Verification items for the finished model (mm, model axes). Give positions to 0.01 mm unless a question says otherwise; leave off trailing zeros. Order: outer loops, then holes, each group sorted by start corner. A loop starts at its lowest first (then second) coordinate and runs counter-clockwise, first axis right, second up. Notation, with made-up numbers: M 34,-12 L 40,-12 A6 ccw 40,-7 Z; hole C 56.25,-22 d7. An arc over 180 degrees is marked long. Answer as a JSON object with one key per item and string values.
```python
from build123d import *

# Parameters (mm, degrees)
F1_DEPTH = 25.4


with BuildPart() as f1:
    # F0 (on Top) → F1 (new body)
    with BuildSketch(Plane.XY):
        with BuildLine():
            Line((-15.537605658, -74.5480572665), (-15.537605658, 74.5990804931))
            ThreePointArc((-15.537605658, 74.5990804931), (-74.5736678483, -15.6591207816), (15.780594342, -74.5480572665))
            Line((15.780594342, -74.5480572665), (-15.537605658, -74.5480572665))
        make_face()
        with BuildLine():
            Line((15.537605658, 74.5990804931), (-15.537605658, 74.5990804931))
            Line((-15.537605658, 74.5990804931), (-15.537605658, -74.5480572665))
            Line((-15.537605658, -74.5480572665), (15.780594342, -74.5480572665))
            Line((15.780594342, -74.5480572665), (15.780594342, 74.5480572665))
            ThreePointArc((15.780594342, 74.5480572665), (15.6591207816, 74.5736678483), (15.537605658, 74.5990804931))
        make_face()
        with BuildLine():
            Line((15.780594342, 74.5480572665), (15.780594342, -74.5480572665))
            ThreePointArc((15.780594342, -74.5480572665), (59.1984851532, -47.9789470036), (76.2, 0))
            ThreePointArc((76.2, 0), (59.1984851532, 47.9789470036), (15.780594342, 74.5480572665))
        make_face()
    extrude(amount=F1_DEPTH)


solid = f1.part
```
Q1. Material ranges on L1, parallel to Y at x = 1, z = 12; L2, parallel to Y at x = 19.5, z = 22; L3, parallel to X at y = 20, z = 9.25, recorded low to high.
Resolved:
{"L1": "y = -76.19 to 74.6", "L2": "y = -73.66 to 73.66", "L3": "x = -73.53 to 73.53"}
Q2. Section check A-A on z = 7.75. Record the cut outline in (x, y), then the cut area to 3 significant figures.
Resolved:
{"outline": "M -15.54,74.6 A76.2 ccw long 15.78,74.55 A76.2 ccw 15.54,74.6 Z", "area": "18,200 mm²"}
Q3. Section check C-C on y = 33. Record the cut outline in (x, z).
Resolved:
{"outline": "M -68.68,0 L 68.68,0 L 68.68,25.4 L -68.68,25.4 Z"}
Q4. Gauge pin test, flat ends, axial feed: pin 1 Ø6 at (x, z) = (-55.5, 15) entering from +Y; pin 2 Ø4 at (x, z) = (56.5, 4) entering from +Y; pin 3 Ø10 at (x, y) = (-1, -27.5) entering from -Z; pin 4 Ø10 at (y, z) = (-56, 8.5) entering from -X. Record the tip position at first contact, or that the pin passes through.
Resolved:
{"pin 1": "stops at y = 55.23", "pin 2": "stops at y = 53.26", "pin 3": "stops at z = 0", "pin 4": "stops at x = -56.62"}
Q5. Section check B-B on x = 34.5. Record the cut outline in (y, z), then the cut area to 3 significant figures.
Resolved:
{"outline": "M -67.94,0 L 67.94,0 L 67.94,25.4 L -67.94,25.4 Z", "area": "3,450 mm²"}
